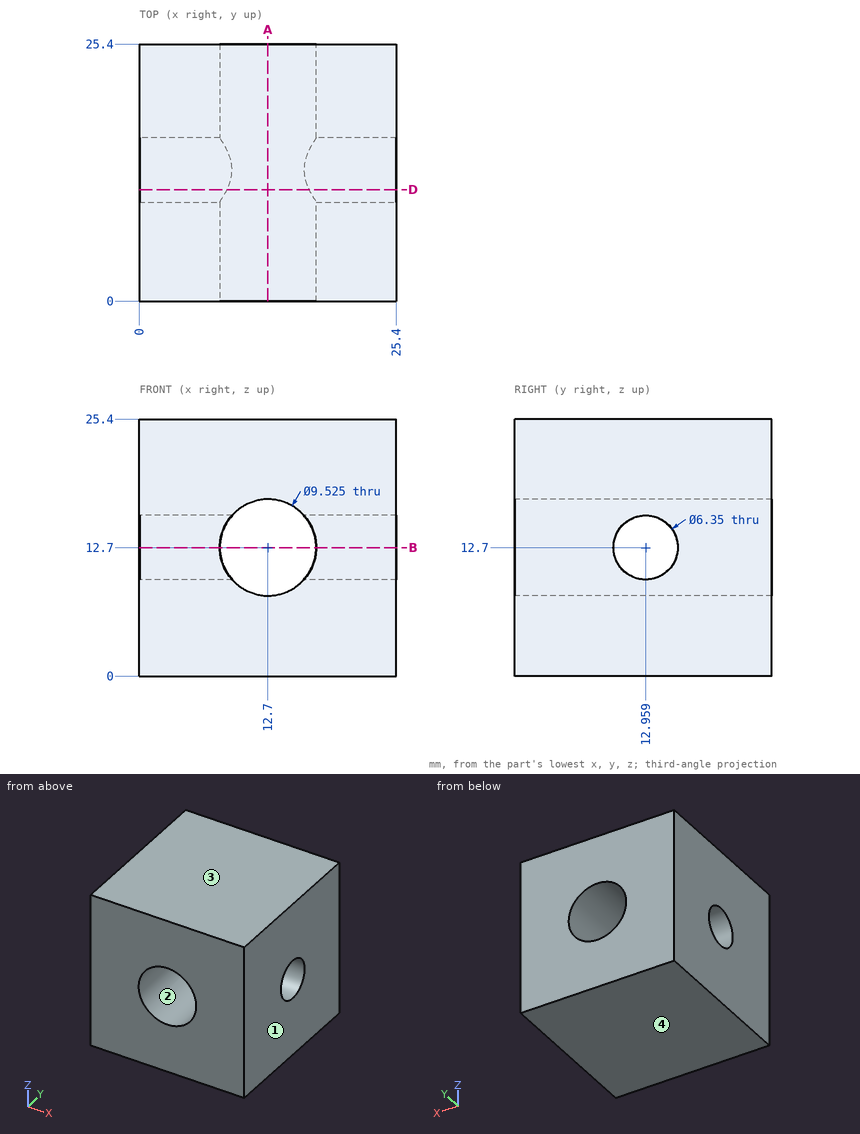
The drawing under review shows one solid part. Ordinate dimensions are in mm from its lowest x, y, z. Coordinates: 2 decimals unless noted, no trailing zeros. Order: outer loops, then holes, each group sorted by start corner. A loop starts at its lowest first (then second) coordinate and runs counter-clockwise, first axis right, second up. Notation, with made-up numbers: (7, 30) -> (63, 30) arc R11 cw to (63, 39) -> close; hole circle Ø2 at (36.5, 85.25). An arc over 180 degrees is marked (long way). Return JSON: item names as keys, results as strings.
1. We need section B-B on z = 12.7. Write out the cut boundary in (x, y) (1 decimal).
Answer block:
{"outline": "(0, 0) -> (7.9, 0) -> (7.9, 9.8) -> (0, 9.8) -> close; (0, 16.1) -> (7.9, 16.1) -> (7.9, 25.4) -> (0, 25.4) -> close; (17.5, 0) -> (25.4, 0) -> (25.4, 9.8) -> (17.5, 9.8) -> close; (17.5, 16.1) -> (25.4, 16.1) -> (25.4, 25.4) -> (17.5, 25.4) -> close"}
2. We need section A-A on x = 12.7. Write out the cut boundary in (y, z), and give its area (3 significant figures).
Answer block:
{"outline": "(0, 0) -> (25.4, 0) -> (25.4, 7.94) -> (0, 7.94) -> close; (0, 17.46) -> (25.4, 17.46) -> (25.4, 25.4) -> (0, 25.4) -> close", "area": "403 mm²"}
3. We need section D-D on y = 11. Write out the cut boundary in (x, z) (1 decimal).
Answer block:
{"outline": "(0, 0) -> (25.4, 0) -> (25.4, 10.2) -> (16.8, 10.2) arc R4.8 cw to (8.6, 10.2) -> (0, 10.2) -> close; (0, 15.2) -> (8.6, 15.2) arc R4.8 cw to (16.8, 15.2) -> (25.4, 15.2) -> (25.4, 25.4) -> (0, 25.4) -> close"}
4. The part is to be moulded in two halves that separate along Z. For the marked faces 1, 2, 3 and 4, say which applies: +Z half, -Z half, draft (parallel to the pull), parting line (faces both ways), or undercut.
Answer block:
{"face 1": "draft", "face 2": "undercut", "face 3": "+Z half", "face 4": "-Z half"}
5. For line 1 (Y direction, x = 5.75, z = 12.7) (1 decimal); line 2 (Z direction, x = 12.7, y = 14), list the stretches that pass through material, from the lowest coordinate up. Write a range as from..to.
Answer block:
{"line 1": "0..9.8, 16.1..25.4", "line 2": "0..7.94, 17.46..25.4"}
